```python
from build123d import *

# Parameters (mm, degrees)
SKETCH2_R               = 1
CUT_EXTRUDE1_DEPTH      = 15
CUT_EXTRUDE2_DEPTH      = 26.396850198
CUT_EXTRUDE2_DEPTH_BACK = 26.396850198
SKETCH3_R               = 2.5


with BuildPart() as part:
    # Sketch1 → Revolve1 (revolve)
    with BuildSketch(Plane.XY, mode=Mode.PRIVATE) as revolve1_sk:
        Polygon((0, 3), (0, 0), (20, 0), (20, 7), (4, 7), align=None)
    revolve(revolve1_sk.sketch.rotate(Axis((0, 0, 0), (1, 0, 0)), 90), axis=Axis((0, 0, 0), (1, 0, 0)))

    # Sketch2 → Cut-Extrude1 (cut)
    with BuildSketch(Plane.ZY):
        Circle(SKETCH2_R)
    extrude(amount=-CUT_EXTRUDE1_DEPTH, mode=Mode.SUBTRACT)

    # Sketch3 → Cut-Extrude2 (cut, two sides: drawn at the far end of the back side and taken through both)
    with BuildSketch(Plane.XY.offset(7).offset(-CUT_EXTRUDE2_DEPTH_BACK)):
        with Locations((9, 0)):
            Circle(SKETCH3_R)
    extrude(amount=CUT_EXTRUDE2_DEPTH + CUT_EXTRUDE2_DEPTH_BACK, mode=Mode.SUBTRACT)


solid = part.part
```
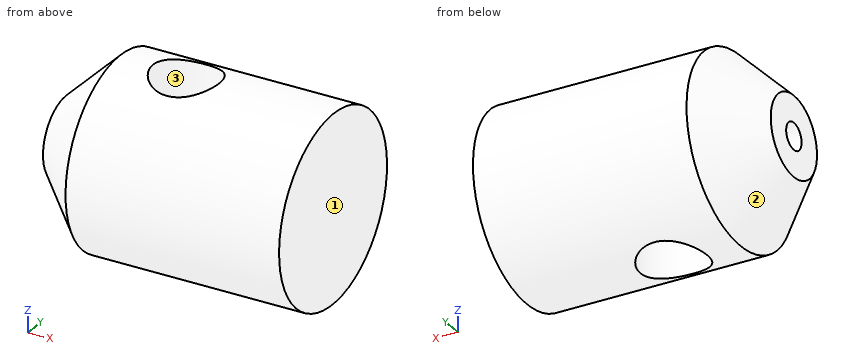
Geometry check sheet. Reference: the model listing, model coordinates, mm. Face numbers are marked on the shaded views. Round coordinates to 2 decimals unless told otherwise and drop trailing zeros. Order: outer loops, then holes, each group sorted by start corner. A loop starts at its lowest first (then second) coordinate and runs counter-clockwise, first axis right, second up. Notation, with made-up numbers: M -26,18 L 4,18 A25 ccw 4,39 Z; hole C 80.5,71 d10. An arc over 180 degrees is marked long. Answer as CSV lines item,"result".
1) Sectioned sample at A-A on y = 0. Record the cut outline in (x, z).
Entries:
outline,"M 0,-3 L 4,-7 L 6.5,-7 L 6.5,-1 L 0,-1 Z; M 0,1 L 6.5,1 L 6.5,7 L 4,7 L 0,3 Z; M 11.5,-7 L 20,-7 L 20,7 L 11.5,7 L 11.5,1 L 15,1 L 15,-1 L 11.5,-1 Z"
2) Thickness scan on probe 1 along Y at (x, z) = (12.9, 0); probe 2 along X at (y, z) = (0, 1.25); probe 3 along X at (y, z) = (-1.5, 4.75). Record the ranges inside material, lowest first. Write a range as [from, to].
Entries:
probe 1,"[-7, -1], [1, 7]"
probe 2,"[0, 6.5], [11.5, 20]"
probe 3,"[1.98, 7], [11, 20]"
3) Sectioned sample at C-C on z = 0. Record the cut outline in (x, y).
Entries:
outline,"M 0,-3 L 4,-7 L 20,-7 L 20,7 L 4,7 L 0,3 L 0,1 L 6.71,1 A2.5 cw 11.29,1 L 15,1 L 15,-1 L 11.29,-1 A2.5 cw 6.71,-1 L 0,-1 Z"
4) Gauge pin test, flat ends, axial feed: pin 1 Ø4 at (x, y) = (9, 0) entering from -Z; pin 2 Ø1.8 at (y, z) = (0, 0) entering from -X; pin 3 Ø1 at (x, y) = (17.5, -4.5) entering from -Z. Record the tip position at first contact, or that the pin passes through.
Entries:
pin 1,"through"
pin 2,"x = 15"
pin 3,"z = -5.74"
5) Sectioned sample at D-D on x = 7.75. Record the cut outline in (y, z), and give its area (3 significant figures).
Entries:
outline,"M -2.17,-6.66 L -2.17,6.66 A7 ccw Z; M 2.17,-6.66 A7 ccw 2.17,6.66 Z"
area,"94.3 mm2"
6) Sectioned sample at B-B on x = 4.75. Record the cut outline in (y, z).
Entries:
outline,"C 0,0 d14; hole C 0,0 d2"
7) Mould release check, pull along X, two halves, no side actions. Record for the marked faces 1, 2 and 3: +X half, -X half, draft (parallel to the pull), parting line (faces both ways), or undercut.
Entries:
face 1,"+X half"
face 2,"-X half"
face 3,"undercut"
